Work out the finished part from the listing and answer in its coordinate system (mm). A direction names the side the tool comes from. Give positions to 0.01 mm unless a question says otherwise; leave off trailing zeros. Order: outer loops, then holes, each group sorted by start corner. A loop starts at its lowest first (then second) coordinate and runs counter-clockwise, first axis right, second up.
```python
from build123d import *

# Parameters (mm, degrees)
BOSS_EXTRUDE1_DEPTH = 5
BOSS_EXTRUDE2_DEPTH = 5
SKETCH4_R           = 9.75
BOSS_EXTRUDE3_DEPTH = 21
BOSS_EXTRUDE4_START = -15
SKETCH5_R           = 13.5
BOSS_EXTRUDE4_DEPTH = 20
SKETCH5_3_R         = 7.25
BOSS_EXTRUDE5_DEPTH = 15
CHAMFER1_SIZE       = 10
CUT_EXTRUDE1_DEPTH  = 10
SKETCH9_R           = 10.15
CUT_EXTRUDE2_DEPTH  = 10
CHAMFER2_SIZE       = 1
SKETCH10_R          = 1.65
CUT_EXTRUDE3_DEPTH  = 32.6785
CIRPATTERN1_COUNT   = 2
CIRPATTERN1_ANGLE   = 90


with BuildPart() as part:
    # Sketch2 → Boss-Extrude1 (new body, symmetric)
    with BuildSketch(Plane.XY):
        with BuildLine():
            ThreePointArc((8.946673347, 36.860907204), (0, 52.857), (-8.946673347, 36.860907204))
            Line((-8.946673347, 36.860907204), (-36.395818719, -10.682407204))
            ThreePointArc((-36.395818719, -10.682407204), (-45.775504768, -26.4285), (-27.449145372, -26.1785))
            Line((-27.449145372, -26.1785), (27.449145372, -26.1785))
            ThreePointArc((27.449145372, -26.1785), (45.775504768, -26.4285), (36.395818719, -10.682407204))
            Line((36.395818719, -10.682407204), (8.946673347, 36.860907204))
        make_face()
        Polygon((-28.02198399, -16.1785), (0, 32.357), (28.02198399, -16.1785), align=None, mode=Mode.SUBTRACT)
    extrude(amount=BOSS_EXTRUDE1_DEPTH, both=True)

    # Sketch3 → Boss-Extrude2 (add)
    with BuildSketch(Plane.XY):
        with BuildLine():
            Line((-16.510991995, 3.759122981), (-11.510991995, 12.419377019))
            ThreePointArc((-11.510991995, 12.419377019), (0, 10.282645658), (11.510991995, 12.419377019))
            Line((11.510991995, 12.419377019), (16.510991995, 3.759122981))
            ThreePointArc((16.510991995, 3.759122981), (8.905032358, -5.141322829), (5, -16.1785))
            Line((5, -16.1785), (-5, -16.1785))
            ThreePointArc((-5, -16.1785), (-8.905032358, -5.141322829), (-16.510991995, 3.759122981))
        make_face()
    extrude(amount=-BOSS_EXTRUDE2_DEPTH)

    # Sketch4 → Boss-Extrude3 (add)
    with BuildSketch(Plane.XY.offset(5)):
        with Locations((-36.682238028, -21.1785)):
            Circle(SKETCH4_R)
        with Locations((36.682238028, -21.1785)):
            Circle(SKETCH4_R)
        with Locations((0, 42.357)):
            Circle(SKETCH4_R)
    extrude(amount=BOSS_EXTRUDE3_DEPTH)

    # Sketch5 → Boss-Extrude4 (add)
    with BuildSketch(Plane.XY.offset(BOSS_EXTRUDE4_START)):
        Circle(SKETCH5_R)
    extrude(amount=BOSS_EXTRUDE4_DEPTH)

    # Sketch5_3 → Boss-Extrude5 (add)
    with BuildSketch(Plane.XY):
        Circle(SKETCH5_3_R)
    extrude(amount=BOSS_EXTRUDE5_DEPTH)

    # Chamfer1
    chamfer1_edges = [part.edges().sort_by_distance(p)[0] for p in [
        (28.02198399, -16.1785, 0),
        (-28.02198399, -16.1785, 0),
        (0, 32.357, 0),
    ]]
    chamfer(chamfer1_edges, length=CHAMFER1_SIZE)

    # Sketch8 → Cut-Extrude1 (cut)
    with BuildSketch(Plane.XY.offset(26)):
        Polygon((-41.682238028, -24.065251346), (-36.682238028, -26.952002692), (-31.682238028, -24.065251346), (-31.682238028, -18.291748654), (-36.682238028, -15.404997308), (-41.682238028, -18.291748654), align=None)
        Polygon((41.682238028, -24.065251346), (41.682238028, -18.291748654), (36.682238028, -15.404997308), (31.682238028, -18.291748654), (31.682238028, -24.065251346), (36.682238028, -26.952002692), align=None)
        Polygon((0, 48.130502692), (-5, 45.243751346), (-5, 39.470248654), (0, 36.583497308), (5, 39.470248654), (5, 45.243751346), align=None)
    extrude(amount=-CUT_EXTRUDE1_DEPTH, mode=Mode.SUBTRACT)

    # Sketch9 → Cut-Extrude2 (cut)
    with BuildSketch(Plane(origin=(0, 0, -15), x_dir=(-1, 0, 0), z_dir=(0, 0, -1))):
        Circle(SKETCH9_R)
    extrude(amount=-CUT_EXTRUDE2_DEPTH, mode=Mode.SUBTRACT)

    # Chamfer2
    chamfer2_edges = [part.edges().sort_by_distance(p)[0] for p in [
        (10.15, 0, -15),
        (-13.5, 0, -15),
    ]]
    chamfer(chamfer2_edges, length=CHAMFER2_SIZE)

    # Sketch10 → Cut-Extrude3 (cut, through all)
    with BuildSketch(Plane(origin=(0, 0, 0), x_dir=(1, 0, 0), z_dir=(0, 1, 0))):
        with Locations((0, 10)):
            Circle(SKETCH10_R)
    cut_extrude3 = extrude(amount=-CUT_EXTRUDE3_DEPTH, mode=Mode.SUBTRACT)

    # CirPattern1: Cut-Extrude3 ×2 about axis
    cirpattern1_axis = Axis((0, 0, 43.183766184), (0, 0, -1))
    for i in range(1, CIRPATTERN1_COUNT):
        add(cut_extrude3.rotate(cirpattern1_axis, i * CIRPATTERN1_ANGLE / (CIRPATTERN1_COUNT - 1)), mode=Mode.SUBTRACT)


solid = part.part
```
1. Straight lines are drawn through the part: probe 1 along Y at (x, z) = (-12.15, -10); probe 2 along Z at (x, y) = (-12.05, 0); probe 3 along Z at (x, y) = (-34, -13). For each, find the intervals that lie inside material, in ascending order.
Findings below:
probe 1: y = -5.88 to -1.65, 1.65 to 5.88
probe 2: z = -15 to -11.65, -8.35 to 5
probe 3: z = -5 to 26
2. The part is cut by section A-A (z = -10). Write down the section's boundary in (x, y), then the cut area to 3 significant figures.
Findings below:
outline: (-13.4, -1.65) arc R13.5 ccw to (-1.65, -13.4) - (-1.65, -10.01) arc R10.15 cw to (-10.01, -1.65) - close; (-13.4, 1.65) - (-10.01, 1.65) arc R10.15 cw (long way) to (1.65, -10.01) - (1.65, -13.4) arc R13.5 ccw (long way) to start
area: 227 mm2
3. The mould has two halves that part along X. Classify faces 1 (the face through (4.499, 33.707, 15.353)), 2 (the face through (-9.582, 11.747, -2.465)), 3 (the face through (-4, -14, -5)): pulls with the +X half, pulls with the -X half, needs draft (parallel to the pull), parting line crosses it, or undercut.
Findings below:
face 1: parting line crosses it
face 2: undercut
face 3: needs draft
4. The part is cut by section C-C (x = 33.5). Write down the section's boundary in (y, z).
Findings below:
outline: (-31.18, -5) - (-5.67, -5) - (-5.67, 5) - (-11.96, 5) - (-11.96, 26) - (-17.24, 26) - (-17.24, 16) - (-25.11, 16) - (-25.11, 26) - (-30.39, 26) - (-30.39, 5) - (-31.18, 5) - close
5. Given P1, Ø16, axis at x = 0, y = 0, coming from the +Z side; P2, Ø2, axis at x = 31.5, z = -3.5, coming from the +Y side; P3, Ø3, axis at y = 9, z = 1.5, coming from the +X side, each flat-ended and moving along its own axis, determine where each tip first touches the part or whether it passes through.
Findings below:
P1: stops at z = 15
P2: stops at y = -0.47
P3: stops at x = 25.9
6. Which of the six approach directions +Z, -Z, +X, -X, +Y, -Y give full straight-line access (tool end or side, diameter ignored) to faces 4 (the face through (39.147, -25.529, 21.07)), 5 (the face through (41, -25, 26)), 6 (the face through (-20.487, -11.909, -0.07)), 7 (the face through (8.05, -6.18, -9.56))?
Findings below:
face 4: +Z
face 5: +Z, +X, -X, +Y, -Y
face 6: +Z, -Z
face 7: -Z
7. The part is cut by section B-B (z = 21.5). State how many separate pieces and enclosed holes the cut face has, then the cut area to 3 significant figures.
Findings below:
separate pieces: 3
enclosed holes: 3
area: 636 mm2
